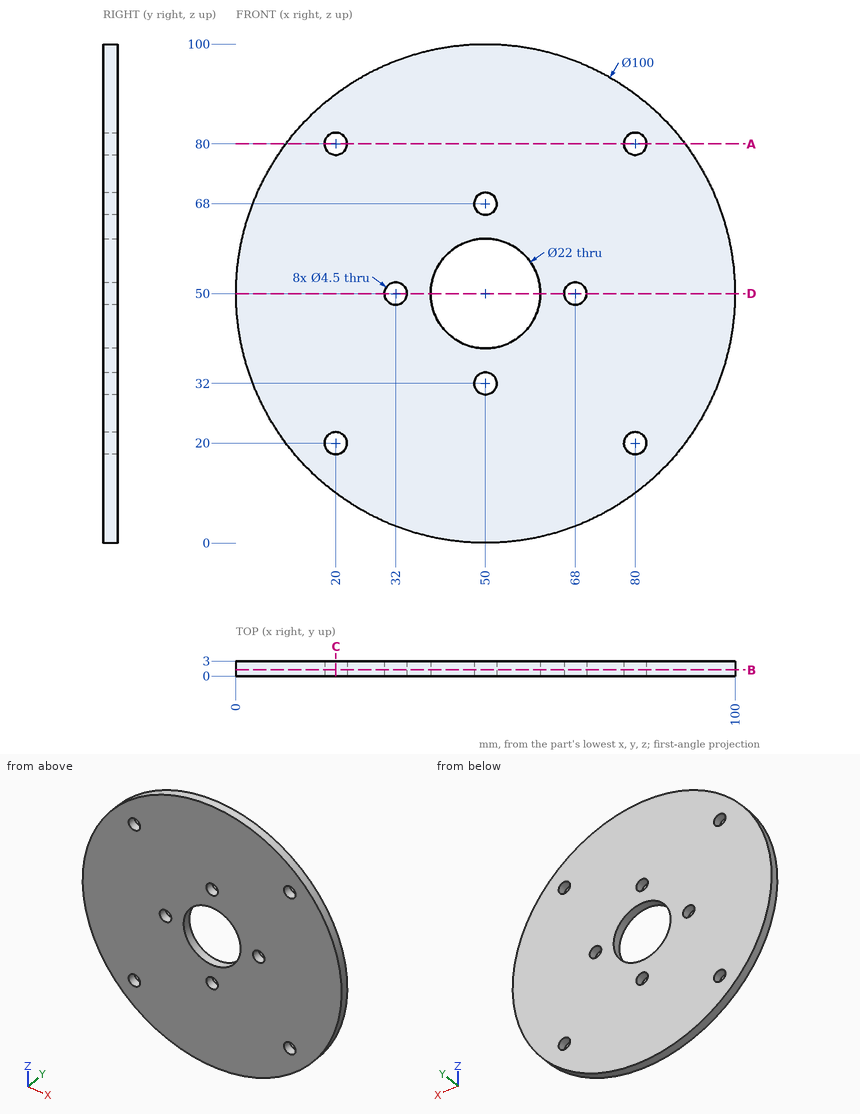
Check sheet for the drawn part. Datum: minimum x, y, z corner. Units: mm. Round coordinates to 2 decimals unless told otherwise and drop trailing zeros. Order: outer loops, then holes, each group sorted by start corner. A loop starts at its lowest first (then second) coordinate and runs counter-clockwise, first axis right, second up. Notation, with made-up numbers: M -16,63 L 23,63 A4 cw 23,67 Z; hole C -33.5,48 d4. An arc over 180 degrees is marked long. Answer in a Markdown table with one row per item.
(1) Material ranges on line 1 along X through (y, z) = (2.2, 50); line 2 along Z through (x, y) = (80, 0.9), recorded low to high. Write a range as from..to.
Findings:
| item | result |
|---|---|
| line 1 | x = 0..29.75, 34.25..39, 61..65.75, 70.25..100 |
| line 2 | z = 10..17.75, 22.25..77.75, 82.25..90 |
(2) Section check C-C on x = 20. Record the boundary of the cut face in (y, z), plus the area to 3 significant figures.
Findings:
| item | result |
|---|---|
| outline | M 0,10 L 3,10 L 3,17.75 L 0,17.75 Z; M 0,22.25 L 3,22.25 L 3,77.75 L 0,77.75 Z; M 0,82.25 L 3,82.25 L 3,90 L 0,90 Z |
| area | 213 mm^2 |
(3) Section check A-A on z = 80. Record the boundary of the cut face in (x, y).
Findings:
| item | result |
|---|---|
| outline | M 10,0 L 17.75,0 L 17.75,3 L 10,3 Z; M 22.25,0 L 77.75,0 L 77.75,3 L 22.25,3 Z; M 82.25,0 L 90,0 L 90,3 L 82.25,3 Z |
(4) Gauge pin test, flat ends, axial feed: pin 1 (7 mm diameter, centred on x = 20, z = 20, fed in from -Y); pin 2 (1.5 mm diameter, centred on x = 14.5, y = 1.5, fed in from -Z). Record the tip position at first contact, or that the pin passes through.
Findings:
| item | result |
|---|---|
| pin 1 | stops at y = 0 |
| pin 2 | stops at z = 14.05 |
(5) Section check D-D on z = 50. Record the boundary of the cut face in (x, y).
Findings:
| item | result |
|---|---|
| outline | M 0,0 L 29.75,0 L 29.75,3 L 0,3 Z; M 34.25,0 L 39,0 L 39,3 L 34.25,3 Z; M 61,0 L 65.75,0 L 65.75,3 L 61,3 Z; M 70.25,0 L 100,0 L 100,3 L 70.25,3 Z |
(6) Section check B-B on y = 1.25. Give the number of separate pieces and of enclosed holes in the cut face, plus the area to 3 significant figures.
Findings:
| item | result |
|---|---|
| separate pieces | 1 |
| enclosed holes | 9 |
| area | 7,350 mm^2 |
